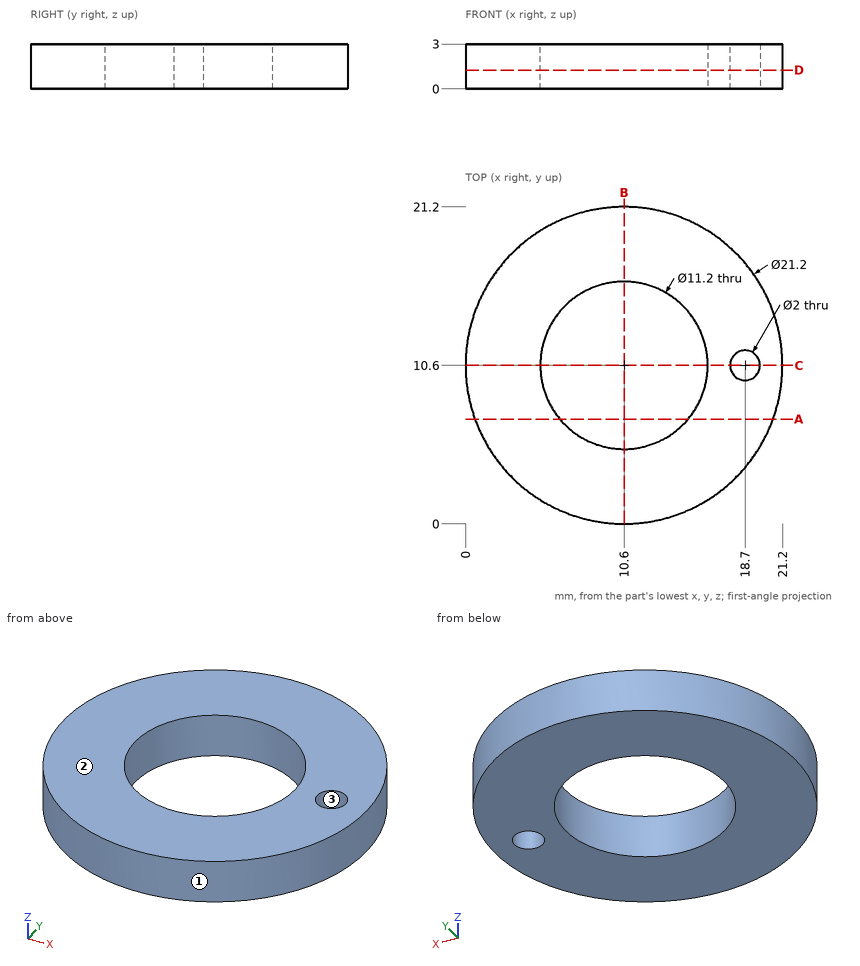
Check sheet for the drawn part. Datum: minimum x, y, z corner. Units: mm. Give positions to 0.01 mm unless a question says otherwise; leave off trailing zeros. Order: outer loops, then holes, each group sorted by start corner. A loop starts at its lowest first (then second) coordinate and runs counter-clockwise, first axis right, second up.
1. Sectioned sample at B-B (x = 10.6). Record the boundary of the cut face in (y, z).
Completed:
outline: (0, 0) - (5, 0) - (5, 3) - (0, 3) - close; (16.2, 0) - (21.2, 0) - (21.2, 3) - (16.2, 3) - close
2. Draft check along X on the marked faces 1, 2 and 3. Enter one of: pulls with the +X half, pulls with the -X half, needs draft (parallel to the pull), parting line crosses it, or undercut.
Completed:
face 1: parting line crosses it
face 2: needs draft
face 3: undercut
3. Sectioned sample at A-A (y = 7). Record the boundary of the cut face in (x, z), then the cut area to 3 significant figures.
Completed:
outline: (0.63, 0) - (6.31, 0) - (6.31, 3) - (0.63, 3) - close; (14.89, 0) - (20.57, 0) - (20.57, 3) - (14.89, 3) - close
area: 34.1 mm2
4. Scan lines: line 1 (Y direction, x = 10.6, z = 0.6); line 2 (X direction, y = 11.25, z = 2.55); line 3 (Y direction, x = 15, z = 0.65). Record each from-to range of solid material in increasing order.
Completed:
line 1: y = 0 to 5, 16.2 to 21.2
line 2: x = 0.02 to 5.04, 16.16 to 17.94, 19.46 to 21.18
line 3: y = 0.96 to 7.14, 14.06 to 20.24
5. Sectioned sample at C-C (y = 10.6). Record the boundary of the cut face in (x, z).
Completed:
outline: (0, 0) - (5, 0) - (5, 3) - (0, 3) - close; (16.2, 0) - (17.7, 0) - (17.7, 3) - (16.2, 3) - close; (19.7, 0) - (21.2, 0) - (21.2, 3) - (19.7, 3) - close
6. Depth check by flat-ended pin: pin 1 (2.5 mm diameter, centred on x = 18.7, y = 10.6, fed in from +Z). Enter the tip coordinate at first touch or a pass-through.
Completed:
pin 1: stops at z = 3
7. Sectioned sample at D-D (z = 1.25). Record the boundary of the cut face in (x, y).
Completed:
outline: circle Ø21.2 at (10.6, 10.6); hole circle Ø11.2 at (10.6, 10.6); hole circle Ø2 at (18.7, 10.6)
